CAD build for the part. Positions are in the model's coordinates, mm. A direction names the side the tool comes from. Give positions to 0.01 mm unless a question says otherwise; leave off trailing zeros. Put each result on its own line as item: value. Start each with the question number.
1. Tool access for faces 4 (the flat face through (9.445, -1.726, -2.471)), 5 (the cylindrical face through (-2.5, -1.7, 14)), 6 (the flat face through (5, -2, 19.428)): list every direction of +Z, -Z, +X, -X, +Y, -Y with a clear straight run to the whole face (end or side of a thin tool).
2. Mould opens along X. For faces 1 (the flat face through (-1, -3.5, 1)), 2 (the flat face through (16.188, -1.726, 12.368)), 3 (the flat face through (4, -2, 16.538)) say: +X half, -X half, draft (parallel to the pull), parting line (faces both ways), or undercut.
3. Cut at A-A on y = -2.65. Give the number of separate pieces and of enclosed holes in the cut face, and give its area (3 significant figures).
4. Wall check: line 1 (X direction, y = -2.65, z = -6); line 2 (X direction, y = -1, z = 14.5); line 3 (X direction, y = -0.95, z = -10). Give the ranges that are in metal, low to high.
5. Drop flat-ended pins along their axis: pin 1 (8 mm diameter, centred on x = -15, z = 15.5, fed in from +Y) (3 decimals); pin 2 (1.8 mm diameter, centred on x = -13.5, y = -1.5, fed in from +Z); pin 3 (1 mm diameter, centred on x = 5.5, y = -2.5, fed in from -Z). Give the stop position or say it passes through.
from build123d import *

# Parameters (mm, degrees)
F1_DEPTH = 3.5


with BuildPart() as f1:
    # F0 (on Front) → F1 (new body)
    with BuildSketch(Plane.XZ):
        with BuildLine():
            Line((11.111137, 19.428022), (-0.664115, 19.428022))
            add(Edge.make_bspline(
                [(-0.664115, 19.428022), (-7.776919, 17.012886), (-18.978179, 6.115542), (-22.016576, -6.739209)],
                knots=[0, 0, 0, 0, 33.773533, 33.773533, 33.773533, 33.773533], degree=3))
            add(Edge.make_bspline(
                [(-22.016576, -6.739209), (-22.068911, -8.466247), (-23.326607, -9.983946), (-19.60919, -12.96701)],
                knots=[0, 0, 0, 0, 6.676901, 6.676901, 6.676901, 6.676901], degree=3))
            add(Edge.make_bspline(
                [(-19.60919, -12.96701), (-12.502755, -15.554382), (-5.717248, -17.509151), (1.972557, -18.273501)],
                knots=[0, 0, 0, 0, 22.22455, 22.22455, 22.22455, 22.22455], degree=3))
            add(Edge.make_bspline(
                [(1.972557, -18.273501), (3.454669, -18.725327), (4.548717, -17.823574), (4.177886, -16.095417)],
                knots=[0, 0, 0, 0, 3.099601, 3.099601, 3.099601, 3.099601], degree=3))
            Line((4.177886, -16.095417), (-0.454777, -3.180466))
            ThreePointArc((-0.454777, -3.180466), (2.403419, 2.858196), (8.442081, 0))
            Line((8.442081, 0), (10.477334, -5.011199))
            add(Edge.make_bspline(
                [(21.124166, -7.553054), (20.007996, -10.873632), (12.419499, -8.047571), (10.477334, -5.011199)],
                knots=[0, 0, 0, 0, 10.946052, 10.946052, 10.946052, 10.946052], degree=3))
            Line((21.124166, -7.553054), (21.124166, 5.503655))
            Line((21.124166, 5.503655), (11.111137, 19.428022))
        make_face()
        with BuildLine():
            ThreePointArc((-16.730794, -11.07734), (-19.449372, -8.358763), (-16.730794, -5.640186))
            Line((-16.730794, -5.640186), (-9.639258, -5.640186))
            ThreePointArc((-9.639258, -5.640186), (-6.920681, -8.358763), (-9.639258, -11.07734))
            Line((-9.639258, -11.07734), (-16.730794, -11.07734))
        make_face(mode=Mode.SUBTRACT)
        with BuildLine():
            ThreePointArc((0, 11.537572), (-2.5, 14.037572), (0, 16.537572))
            Line((0, 16.537572), (7.50006, 16.537572))
            ThreePointArc((7.50006, 16.537572), (10.00006, 14.037572), (7.50006, 11.537572))
            Line((7.50006, 11.537572), (0, 11.537572))
        make_face(mode=Mode.SUBTRACT)
    extrude(amount=F1_DEPTH)


solid = f1.part
Report:
1. face 4: -Z, +Y, -Y
1. face 5: +Y, -Y
1. face 6: +Z, +X, -X, +Y, -Y
2. face 1: draft
2. face 2: +X half
2. face 3: undercut
3. separate pieces: 1
3. enclosed holes: 2
3. area: 898 mm²
4. line 1: x = -21.83 to -18.08, -8.29 to 0.56, 11.31 to 21.12
4. line 2: x = -8.6 to -2.46, 9.96 to 14.65
4. line 3: x = -22.07 to -18.9, -7.47 to 1.99
5. pin 1: passes through
5. pin 2: stops at z = 10.56
5. pin 3: stops at z = 2.69
